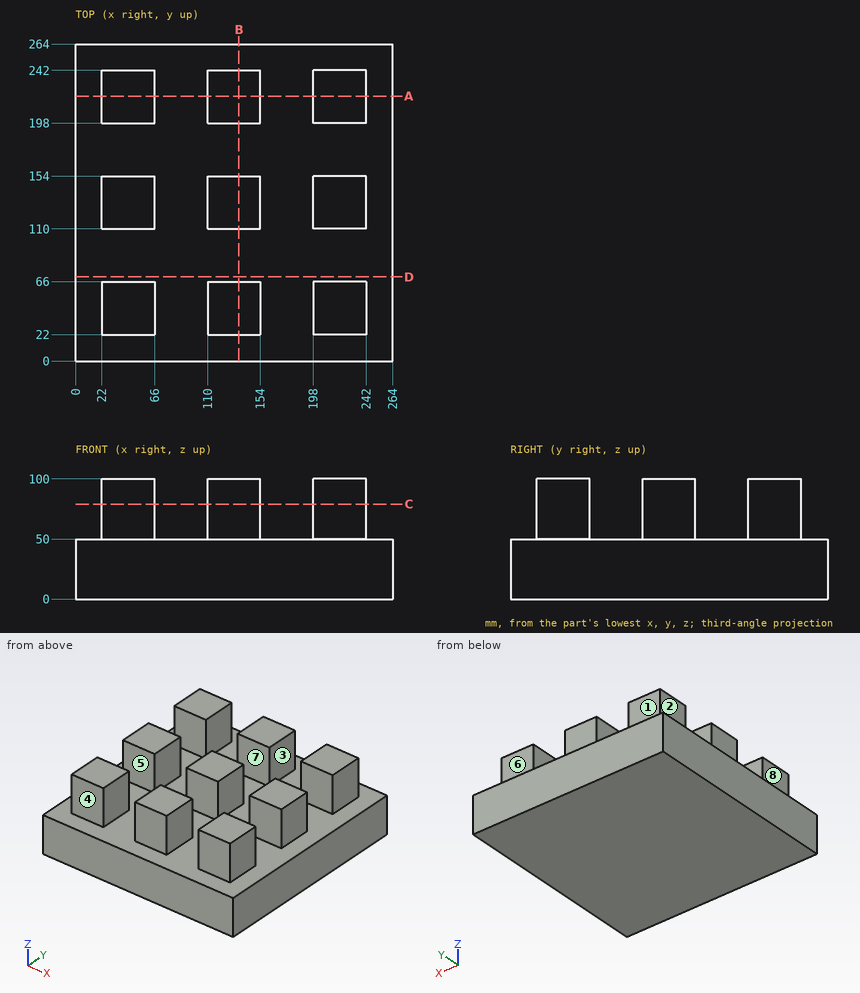
Answer from the drawing. Dimensions are ordinates in mm from the lowest x, y and z of the part. A direction names the side the tool comes from. Round coordinates to 2 decimals unless told otherwise and drop trailing zeros. Loops run counter-clockwise (first coordinate to the right, second up) from the corner with the lowest first, then second, coordinate; pieces in that order, holes last. Notation, with made-up numbers: (45, 67) - (99, 67) arc R23 cw to (99, 82) - close; hole circle Ø2 at (31.25, 3). An arc over 180 degrees is marked (long way). One line per item, written item: value.
Q1. Each of these flat-tipped pins is pushed along its axis until it touches: pin 1 Ø22 at (y, z) = (142.5, 82.5) entering from +X; pin 2 Ø13 at (y, z) = (211, 86.5) entering from -X; pin 3 Ø22 at (x, z) = (221, 83) entering from +Y. Where does it stop, or does it pass through?
Check values:
pin 1: x = 242
pin 2: x = 22
pin 3: y = 242
Q2. The mould has two halves that part along Y. Classify the marked faces 5, 6, 7 and 8: +Y half, -Y half, draft (parallel to the pull), parting line (faces both ways), or undercut.
Check values:
face 5: undercut
face 6: +Y half
face 7: undercut
face 8: draft
Q3. Find section C-C on z = 79. State how many separate pieces and enclosed holes the cut face has, and give its area (3 significant figures).
Check values:
separate pieces: 9
enclosed holes: 0
area: 17,400 mm2
Q4. Straight lines are drawn through the part: probe 1 along X at (y, z) = (125.5, 88); probe 2 along Z at (x, y) = (84.5, 194). For each, find the intervals that lie inside material, in ascending order.
Check values:
probe 1: 22 to 66, 110 to 154, 198 to 242
probe 2: 0 to 50
Q5. Find section D-D on y = 70. Give the vertices of the cut face in (x, z).
Check values:
outline: (0, 0) - (264, 0) - (264, 50) - (0, 50) - close
Q6. For the marked faces 1, 2, 3 and 4, determine the directions among +Z, -Z, +X, -X, +Y, -Y from which every point of the face is accessible in a straight line to the end or side of a thin tool.
Check values:
face 1: +Z, +X, -X, +Y
face 2: +Z, -X, +Y, -Y
face 3: +Z, +Y, -Y
face 4: +Z, +X, -X, -Y
Q7. Find section A-A on y = 220.5. Give the vertices of the cut face in (x, z), and give its area (3 significant figures).
Check values:
outline: (0, 0) - (264, 0) - (264, 50) - (242, 50) - (242, 100) - (198, 100) - (198, 50) - (154, 50) - (154, 100) - (110, 100) - (110, 50) - (66, 50) - (66, 100) - (22, 100) - (22, 50) - (0, 50) - close
area: 19,800 mm2
